The listing builds one solid part. Answer for the finished solid, in the listing's coordinates (mm). Face numbers are marked on the shaded views. A direction names the side the tool comes from. Coordinates: 2 decimals unless noted, no trailing zeros. Loops run counter-clockwise (first coordinate to the right, second up) from the corner with the lowest first, then second, coordinate; pieces in that order, holes last. Notation, with made-up numbers: (60.25, -16) - (83.25, -16) arc R24 ccw to (83.25, 14) - close; hole circle Ø4 at (-32, 58.5). An arc over 180 degrees is marked (long way). Use one line per item in the form item = value. Start each with the question number.
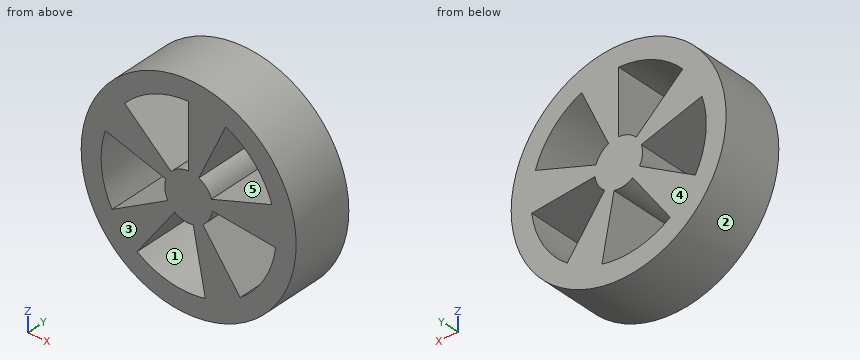
```python
from build123d import *

# Parameters (mm, degrees)
F0_R     = 6.75
F1_DEPTH = 4
F3_DEPTH = 25


with BuildPart() as f1:
    # F0 (on Front) → F1 (new body)
    with BuildSketch(Plane.XZ):
        Circle(F0_R)
    extrude(amount=F1_DEPTH)

    # F2 (on face) → F3 (cut)
    with BuildSketch(Plane.XZ.offset(4)):
        with BuildLine():
            Line((0, 1.5), (0, 5.5))
            ThreePointArc((0, 5.5), (-2.19312, 5.04383), (-4.022445, 3.750991))
            Line((-4.022445, 3.750991), (-1.097031, 1.022998))
            ThreePointArc((-1.097031, 1.022998), (-0.598124, 1.37559), (0, 1.5))
        make_face()
        with BuildLine():
            Line((1.426585, 0.463525), (5.230811, 1.699593))
            ThreePointArc((5.230811, 1.699593), (4.119256, 3.64441), (2.3244, 4.984693))
            Line((2.3244, 4.984693), (0.633927, 1.359462))
            ThreePointArc((0.633927, 1.359462), (1.123434, 0.99393), (1.426585, 0.463525))
        make_face()
        with BuildLine():
            ThreePointArc((3.232819, -4.449593), (4.73896, -2.791461), (5.459004, -0.670281))
            Line((5.459004, -0.670281), (1.488819, -0.182804))
            ThreePointArc((1.488819, -0.182804), (1.292444, -0.761308), (0.881678, -1.213525))
            Line((0.881678, -1.213525), (3.232819, -4.449593))
        make_face()
        with BuildLine():
            ThreePointArc((-3.232819, -4.449593), (-1.190418, -5.369628), (1.049449, -5.39895))
            Line((1.049449, -5.39895), (0.286213, -1.472441))
            ThreePointArc((0.286213, -1.472441), (-0.324659, -1.464444), (-0.881678, -1.213525))
            Line((-0.881678, -1.213525), (-3.232819, -4.449593))
        make_face()
        with BuildLine():
            Line((-1.426585, 0.463525), (-5.230811, 1.699593))
            ThreePointArc((-5.230811, 1.699593), (-5.474679, -0.527152), (-4.810408, -2.666453))
            Line((-4.810408, -2.666453), (-1.31193, -0.727214))
            ThreePointArc((-1.31193, -0.727214), (-1.493094, -0.143769), (-1.426585, 0.463525))
        make_face()
    extrude(amount=-F3_DEPTH, mode=Mode.SUBTRACT)


solid = f1.part
```
(1) Find the intervals of material crossed by probe 1 along Z at (x, y) = (2.25, -2.55); probe 2 along Z at (x, y) = (4, -1.4); probe 3 along X at (y, z) = (-3.55, 4.25), in increasing order. Write a range as from..to.
(2) A cutting plane is placed at A-A (z = 0). Determine the outline of the cut face in (x, y), then the cut area to 3 significant figures.
(3) Each of these flat-tipped pins is pushed along its axis until it touches: pin 1 Ø1 at (x, y) = (4, -1) entering from -Z; pin 2 Ø1 at (x, y) = (-5, -0.5) entering from +Z; pin 3 Ø1.5 at (x, y) = (4.5, -1) entering from +Z. Where does it stop, or does it pass through?
(4) For the marked faces 4 and 5, determine the directions among +Z, -Z, +X, -X, +Y, -Y from which every point of the face is accessible in a straight line to the end or side of a thin tool.
(5) A cutting plane is placed at D-D (z = -2.5). Determine the outline of the cut face in (x, y), then the cut area to 3 significant figures.
(6) A cutting plane is placed at B-B (x = 4.5). Determine the outline of the cut face in (y, z), then the cut area to 3 significant figures.
(7) A cutting plane is placed at C-C (y = -2.9). Determine the outline of the cut face in (x, z), then the cut area to 3 significant figures.
(8) Determine the mould class of the marked faces 1, 2 and 3 for opening direction Z: +Z half, -Z half, draft (parallel to the pull), parting line (faces both ways), or undercut.
Evaluation:
q1.probe_1 = -6.36..-3.1, -0.28..0.73, 4.83..6.36
q1.probe_2 = -5.44..-3.77, -0.49..1.3, 3.77..5.44
q1.probe_3 = -5.24..-3.49, 0..1.98, 3.49..5.24
q2.outline = (-6.75, -4) - (-5.5, -4) - (-5.5, 0) - (-6.75, 0) - close; (-1.5, -4) - (6.75, -4) - (6.75, 0) - (-1.5, 0) - close
q2.area = 38.0 mm^2
q3.pin_1 = -5.77
q3.pin_2 = 5.03
q3.pin_3 = 5.61
q4.face_4 = +Z, -Z, +X, -X, +Y
q4.face_5 = +Y, -Y
q5.outline = (-6.27, -4) - (-4.9, -4) - (-4.9, 0) - (-6.27, 0) - close; (-4.51, -4) - (-1.82, -4) - (-1.82, 0) - (-4.51, 0) - close; (0.49, -4) - (1.82, -4) - (1.82, 0) - (0.49, 0) - close; (4.9, -4) - (6.27, -4) - (6.27, 0) - (4.9, 0) - close
q5.area = 27.1 mm^2
q6.outline = (-4, -5.03) - (0, -5.03) - (0, -3.16) - (-4, -3.16) - close; (-4, -0.55) - (0, -0.55) - (0, 1.46) - (-4, 1.46) - close; (-4, 3.16) - (0, 3.16) - (0, 5.03) - (-4, 5.03) - close
q6.area = 23.0 mm^2
q7.outline = circle Ø13.5 at (0, 0); hole (-5.23, 1.7) arc R5.5 ccw to (-4.81, -2.67) - (-1.31, -0.73) arc R1.5 cw to (-1.43, 0.46) - close; hole (-4.02, 3.75) - (-1.1, 1.02) arc R1.5 cw to (0, 1.5) - (0, 5.5) arc R5.5 ccw to start; hole (-3.23, -4.45) arc R5.5 ccw to (1.05, -5.4) - (0.29, -1.47) arc R1.5 cw to (-0.88, -1.21) - close; hole (0.63, 1.36) arc R1.5 cw to (1.43, 0.46) - (5.23, 1.7) arc R5.5 ccw to (2.32, 4.98) - close; hole (0.88, -1.21) - (3.23, -4.45) arc R5.5 ccw to (5.46, -0.67) - (1.49, -0.18) arc R1.5 cw to start
q7.area = 85.7 mm^2
q8.face_1 = undercut
q8.face_2 = parting line
q8.face_3 = draft
